```python
from build123d import *

# Parameters (mm, degrees)
F0_R     = 1.5
F1_DEPTH = 5


# Not quite as in the source:
# - a feature names something its author has since deleted; it is built from what else it names


with BuildPart() as f1:
    # F0 (on Top) → F1 (new body)
    with BuildSketch(Plane.XY):
        with BuildLine():
            ThreePointArc((-53.3961581093, 110.9291565406), (-63.4156131399, 113.1914108601), (-68.8598231895, 104.4811955556))
            add(Edge.make_bspline(
                [(-63.2980641383, 107.0343052721), (-66.1125104261, 105.8114732046), (-68.8598231895, 104.4811955556)],
                knots=[2.0399471573, 2.0399471573, 2.0399471573, 2.0850163371, 2.0850163371, 2.0850163371], degree=2, weights=[1, 0.9997461069, 1]))
            ThreePointArc((-63.2980641383, 107.0343052721), (-61.4906892533, 108.5767961292), (-59.1228145122, 108.7744099698))
            add(Edge.make_bspline(
                [(-53.3961581093, 110.9291565406), (-56.2875684522, 109.9066162001), (-59.1228145122, 108.7744099698)],
                knots=[1.962107852, 1.962107852, 1.962107852, 2.0067839239, 2.0067839239, 2.0067839239], degree=2, weights=[1, 0.9997505164, 1]))
        make_face()
        with BuildLine():
            add(Edge.make_bspline(
                [(-63.2980641383, 107.0343052721), (-66.1125104261, 105.8114732046), (-68.8598231895, 104.4811955556)],
                knots=[2.0399471573, 2.0399471573, 2.0399471573, 2.0850163371, 2.0850163371, 2.0850163371], degree=2, weights=[1, 0.9997461069, 1]))
            ThreePointArc((-68.8598231895, 104.4811955556), (-59.7404868081, 96.128795014), (-51.125, 105))
            ThreePointArc((-51.125, 105), (-51.7122161654, 108.1746281846), (-53.3961581093, 110.9291565406))
            add(Edge.make_bspline(
                [(-53.3961581093, 110.9291565406), (-56.2875684522, 109.9066162001), (-59.1228145122, 108.7744099698)],
                knots=[1.962107852, 1.962107852, 1.962107852, 2.0067839239, 2.0067839239, 2.0067839239], degree=2, weights=[1, 0.9997505164, 1]))
            ThreePointArc((-59.1228145122, 108.7744099698), (-56.9656369066, 107.4100343602), (-56.125, 105))
            ThreePointArc((-56.125, 105), (-61.0572668689, 101.2720230999), (-63.2980641383, 107.0343052721))
        make_face()
        with BuildLine():
            add(Edge.make_bspline(
                [(-68.8598231895, 104.4811955556), (-140, 70.0343759485), (-140, 0)],
                knots=[2.0850163371, 2.0850163371, 2.0850163371, 3.1415926536, 3.1415926536, 3.1415926536], degree=2, weights=[1, 0.863671199, 1]))
            Line((-140, 0), (-110, 0))
            add(Edge.make_bspline(
                [(110, 0), (110, 90), (0, 90), (-110, 90), (-110, 0)],
                knots=[0, 0, 0, 1.5707963268, 1.5707963268, 3.1415926536, 3.1415926536, 3.1415926536], degree=2, weights=[1, 0.7071067812, 1, 0.7071067812, 1]))
            Line((110, 0), (140, 0))
            add(Edge.make_bspline(
                [(140, 0), (140, 70.0343759485), (68.8598231895, 104.4811955556)],
                knots=[0, 0, 0, 1.0565763165, 1.0565763165, 1.0565763165], degree=2, weights=[1, 0.863671199, 1]))
            ThreePointArc((68.8598231895, 104.4811955556), (56.5843868601, 96.8085891399), (53.3961581093, 110.9291565406))
            add(Edge.make_bspline(
                [(53.3961581093, 110.9291565406), (0, 129.81257993), (-53.3961581093, 110.9291565406)],
                knots=[1.1794848016, 1.1794848016, 1.1794848016, 1.962107852, 1.962107852, 1.962107852], degree=2, weights=[1, 0.9244096378, 1]))
            ThreePointArc((-53.3961581093, 110.9291565406), (-51.7122161654, 108.1746281846), (-51.125, 105))
            ThreePointArc((-51.125, 105), (-59.7404868081, 96.128795014), (-68.8598231895, 104.4811955556))
        make_face()
        with Locations((-124.0382502632, 13)):
            Circle(F0_R, mode=Mode.SUBTRACT)
        with Locations((-70.333152659, 86.8019097296)):
            Circle(F0_R, mode=Mode.SUBTRACT)
        with Locations((124.0382502632, 13)):
            Circle(F0_R, mode=Mode.SUBTRACT)
        with Locations((0, 105)):
            Circle(F0_R, mode=Mode.SUBTRACT)
        with Locations((70.333152659, 86.8019097296)):
            Circle(F0_R, mode=Mode.SUBTRACT)
        with BuildLine():
            add(Edge.make_bspline(
                [(68.8598231895, 104.4811955556), (66.1125104261, 105.8114732046), (63.2980641383, 107.0343052721)],
                knots=[1.0565763165, 1.0565763165, 1.0565763165, 1.1016454963, 1.1016454963, 1.1016454963], degree=2, weights=[1, 0.9997461069, 1]))
            ThreePointArc((68.8598231895, 104.4811955556), (68.871204986, 104.7404868081), (68.875, 105))
            ThreePointArc((68.875, 105), (63.1746281846, 113.2877838346), (53.3961581093, 110.9291565406))
            add(Edge.make_bspline(
                [(59.1228145122, 108.7744099698), (56.2875684522, 109.9066162001), (53.3961581093, 110.9291565406)],
                knots=[1.1348087297, 1.1348087297, 1.1348087297, 1.1794848016, 1.1794848016, 1.1794848016], degree=2, weights=[1, 0.9997505164, 1]))
            ThreePointArc((59.1228145122, 108.7744099698), (61.4906892533, 108.5767961292), (63.2980641383, 107.0343052721))
        make_face()
        with BuildLine():
            ThreePointArc((53.3961581093, 110.9291565406), (56.5843868601, 96.8085891399), (68.8598231895, 104.4811955556))
            add(Edge.make_bspline(
                [(68.8598231895, 104.4811955556), (66.1125104261, 105.8114732046), (63.2980641383, 107.0343052721)],
                knots=[1.0565763165, 1.0565763165, 1.0565763165, 1.1016454963, 1.1016454963, 1.1016454963], degree=2, weights=[1, 0.9997461069, 1]))
            ThreePointArc((63.2980641383, 107.0343052721), (63.7279769001, 106.0572668689), (63.875, 105))
            ThreePointArc((63.875, 105), (57.5899656398, 101.9656369066), (59.1228145122, 108.7744099698))
            add(Edge.make_bspline(
                [(59.1228145122, 108.7744099698), (56.2875684522, 109.9066162001), (53.3961581093, 110.9291565406)],
                knots=[1.1348087297, 1.1348087297, 1.1348087297, 1.1794848016, 1.1794848016, 1.1794848016], degree=2, weights=[1, 0.9997505164, 1]))
        make_face()
    extrude(amount=F1_DEPTH)


solid = f1.part
```
Build history of the part. All positions in model axes, mm. Coordinates: 2 decimals unless noted, no trailing zeros.
1. Drop flat-ended pins along their axis: pin 1 (3 mm diameter, centred on x = 65, z = 0.5, fed in from -Y); pin 2 (1.5 mm diameter, centred on y = 61.5, z = 1, fed in from -X). Give the stop position or say it passes through.
Answer block:
pin 1: stops at y = 71.69
pin 2: stops at x = -120.73
2. Band-saw the part on A-A, the plane z = 0.85. Give the number of separate pieces and of enclosed holes in the cut face, and give its area (3 significant figures).
Answer block:
separate pieces: 1
enclosed holes: 7
area: 10,800 mm2
3. Pull direction X, two halves, no side cores. Call faces 1 (the cylindrical face through (-63.27, 113.25, 2.46)), 2 (the flat face through (-11, 94, 0)): released by +X, released by -X, zero draft, split by the parting line, or undercut.
Answer block:
face 1: undercut
face 2: zero draft
4. Drill centre lines: probe 1 along X at (y, z) = (105, 1.05) (3 decimals); probe 2 along Y at (x, z) = (60, 1.6) (3 decimals); probe 3 along X at (y, z) = (57, 0.45). Where is each one in solid material? Low to high.
Answer block:
probe 1: x = -68.875 to -63.875, -56.125 to -1.5, 1.5 to 56.125, 63.875 to 68.875
probe 2: y = 75.433 to 101.125, 108.875 to 113.875
probe 3: x = -123.2 to -85.13, 85.13 to 123.2
